For this review, take the finished solid that the model builds, in its own axes (mm). Face numbers are marked on the shaded views. A direction names the side the tool comes from. Give positions to 0.01 mm unless a question says otherwise; leave off trailing zeros. Order: outer loops, then holes, each group sorted by start corner. A loop starts at its lowest first (then second) coordinate and runs counter-clockwise, first axis right, second up. Notation, with made-up numbers: (57, 28) - (90, 28) arc R4 cw to (90, 32) - close; hole circle Ø10 at (-7, 37). An arc over 180 degrees is marked (long way). One line per item, written item: value.
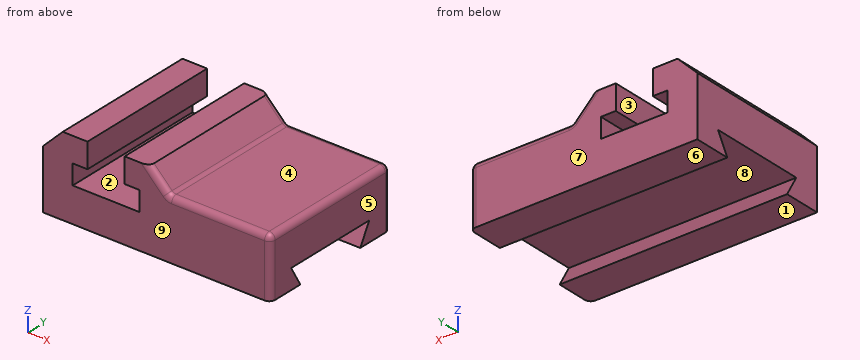
```python
from build123d import *

# Parameters (mm, degrees)
F1_DEPTH = 38.1
F2_R     = 3.048
F4_DEPTH = 116.84


with BuildPart() as f1:
    # F0 (on Front) → F1 (new body, symmetric)
    with BuildSketch(Plane.XZ):
        Polygon((5.08, 10.2046737447), (15.24, 10.2046737447), (5.08, 20.3646737447), align=None)
        Polygon((-49.53, -20.2753262553), (67.31, -20.2753262553), (67.31, 10.2046737447), (15.24, 10.2046737447), (5.08, 10.2046737447), (5.08, 20.3646737447), (-7.62, 20.3646737447), (-7.62, 7.6646737447), (0, 7.6646737447), (0, -2.4953262553), (-34.29, -2.4953262553), (-34.29, 7.6646737447), (-26.67, 7.6646737447), (-26.67, 20.3646737447), (-39.37, 20.3646737447), (-49.53, 10.2046737447), align=None)
    extrude(amount=F1_DEPTH, both=True)

    # F2
    f2_edges = [f1.edges().sort_by_distance(p)[0] for p in [
        (10.16, -38.1, 15.284674),
        (15.24, 0, 10.204674),
        (67.31, -38.1, -5.035326),
        (67.31, 0, 10.204674),
        (41.275, 38.1, 10.204674),
        (67.31, 38.1, -5.035326),
        (10.16, 38.1, 15.284674),
        (41.275, -38.1, 10.204674),
    ]]
    fillet(f2_edges, radius=F2_R)

    # F3 (on face) → F4 (cut)
    with BuildSketch(Plane.YZ.offset(67.31)):
        Polygon((-19.05, -20.2753262553), (0, -20.2753262553), (19.05, -20.2753262553), (19.051521265, -20.2753262553), (24.9174, -10.1153262553), (0, -10.1153262553), (-24.915878735, -10.1153262553), align=None)
    extrude(amount=-F4_DEPTH, mode=Mode.SUBTRACT)


solid = f1.part
```
(1) Take a section at B-B (x = -28). Write out the cut boundary in (y, z).
Answers below:
outline: (-38.1, -20.28) - (-19.05, -20.28) - (-24.92, -10.12) - (24.92, -10.12) - (19.05, -20.28) - (38.1, -20.28) - (38.1, -2.5) - (-38.1, -2.5) - close; (-38.1, 7.66) - (38.1, 7.66) - (38.1, 20.36) - (-38.1, 20.36) - close
(2) Take a section at D-D (x = 24). Write out the cut boundary in (y, z), then the cut area to 3 significant figures.
Answers below:
outline: (-38.1, -20.28) - (-19.05, -20.28) - (-24.92, -10.12) - (24.92, -10.12) - (19.05, -20.28) - (38.1, -20.28) - (38.1, 7.16) arc R3.05 ccw to (35.05, 10.2) - (-35.05, 10.2) arc R3.05 ccw to (-38.1, 7.16) - close
area: 1,870 mm^2
(3) Wall thickness on line 1 (Z direction, x = -3, y = -34.5); line 2 (X direction, y = -15, z = 1); line 3 (Z direction, x = -17, y = 32): over which ranges is each line inside the solid? List them lowest first. Write a range as from..to.
Answers below:
line 1: z = -20.28..-2.5, 7.66..20.36
line 2: x = -49.53..-34.29, 0..67.31
line 3: z = -20.28..-2.5
(4) Draft analysis for pull direction Y (two halves, no side actions). For the marked faces 6, 7, 8 and 9, state which applies: pulls with the +Y half, pulls with the -Y half, needs draft (parallel to the pull), parting line crosses it, or undercut.
Answers below:
face 6: needs draft
face 7: pulls with the +Y half
face 8: undercut
face 9: pulls with the -Y half
(5) Take a section at C-C (y = -3). Write out the cut boundary in (x, z), then the cut area to 3 significant figures.
Answers below:
outline: (-49.53, -10.12) - (67.31, -10.12) - (67.31, 7.16) arc R3.05 ccw to (64.26, 10.2) - (16.5, 10.2) arc R3.05 cw to (14.35, 11.1) - (5.08, 20.36) - (-7.62, 20.36) - (-7.62, 7.66) - (0, 7.66) - (0, -2.5) - (-34.29, -2.5) - (-34.29, 7.66) - (-26.67, 7.66) - (-26.67, 20.36) - (-39.37, 20.36) - (-49.53, 10.2) - close
area: 2,340 mm^2
(6) Take a section at A-A (z = 0.5). Write out the cut boundary in (x, y).
Answers below:
outline: (-49.53, -38.1) - (-34.29, -38.1) - (-34.29, 38.1) - (-49.53, 38.1) - close; (0, -38.1) - (64.26, -38.1) arc R3.05 ccw to (67.31, -35.05) - (67.31, 35.05) arc R3.05 ccw to (64.26, 38.1) - (0, 38.1) - close
(7) Machinability: for the marked faces 1, 2, 3, 4 and 5, which of the approach directions +Z, -Z, +X, -X, +Y, -Y give a long, thin tool a straight path to every point of the face, cutting with its end or side? Answer none if there is none.
Answers below:
face 1: -Z, +X, -X, +Y, -Y
face 2: +Y, -Y
face 3: +Z, +Y, -Y
face 4: +Z, +X, +Y, -Y
face 5: +Z, -Z, +X, +Y, -Y
(8) For P1, Ø2.5, axis at x = -4.5, y = 5, coming from the -Z side; P2, Ø10, axis at y = 17, z = 15.5, coming from the +X side; P3, Ø5, axis at y = 22.5, z = 14, coming from the +X side, all flat-tipped, find the tip position at first contact; note any pin that passes through.
Answers below:
P1: stops at z = -10.12
P2: stops at x = 15.19
P3: stops at x = 13.94
